Can you work these out from the model? Positions are in its coordinate system, mm. Face numbers are marked on the shaded views. A direction names the side the tool comes from. Coordinates: 2 decimals unless noted, no trailing zeros. Loops run counter-clockwise (first coordinate to the right, second up) from the corner with the lowest first, then second, coordinate; pieces in that order, holes last. Notation, with made-up numbers: M 15.25,-5.75 L 24.25,-5.75 A17 cw 24.25,13.25 Z; hole C 84,49 d9. An arc over 180 degrees is marked long. Answer as a JSON object with one key per item and string values. Group by question number.
Item 1: I'm going to push a flat-ended pin straight in: pin 1 Ø7 at (x, z) = (13, -0.5) entering from +Y. Where does the tip first touch, or does it pass through?
Item 2: Suppose I cut it at A-A (y = 19.54). Write out the boundary of the cut face in (x, z).
Item 3: Which directions (+Z, -Z, +X, -X, +Y, -Y) give clear straight access to the entire face, cutting with the end or side of a thin tool? Please do the marked faces 1 and 2.
Item 4: Suppose I cut it at B-B (x = 0). Write out the boundary of the cut face in (y, z).
Item 5: Suppose I cut it at D-D (y = 12). Write out the boundary of the cut face in (x, z), then the cut area to 3 significant figures.
Item 6: Suppose I cut it at C-C (y = 30.04). Count the separate pieces of the cut face and the enclosed holes in it, then the cut area to 3 significant figures.
Item 7: If I drill on line 1 (Z direction, x = -29, y = 30); line 2 (X direction, y = 12, z = -4.75); line 3 (Y direction, x = -11, z = -6), over which ranges is the centre line in solid material (lowest first)?
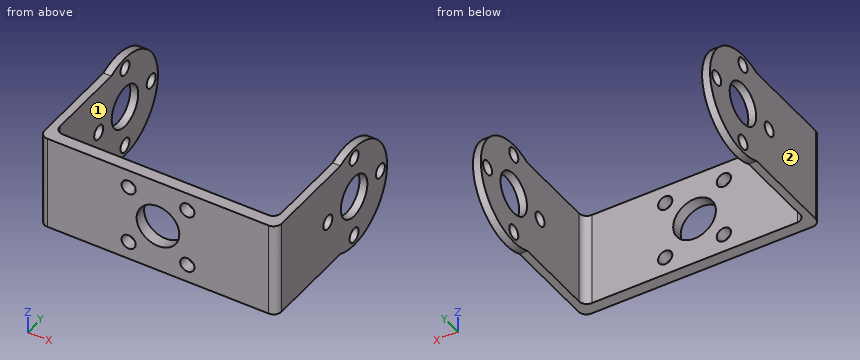
```python
from build123d import *

# Parameters (mm, degrees)
CROQUIS1_W              = 60
CROQUIS1_H              = 24
SALIENTE_EXTRUIR1_DEPTH = 2
CROQUIS3_R              = 5.3
SALIENTE_EXTRUIR2_DEPTH = 2
CROQUIS5_R              = 1.8
CORTAR_EXTRUIR1_DEPTH   = 2
CROQUIS6_W              = 60
CROQUIS6_H              = 24
SALIENTE_EXTRUIR3_DEPTH = 1
CORTAR_EXTRUIR2_REACH   = 46.22
CROQUIS7_R              = 5.4
CROQUIS7_R_2            = 1.8
REDONDEO1_R             = 2


with BuildPart() as part:
    # Croquis1 → Saliente-Extruir1 (new body)
    with BuildSketch(Plane(origin=(0, 0, 0), x_dir=(1, 0, 0), z_dir=(0, 1, 0))):
        Rectangle(CROQUIS1_W, CROQUIS1_H)
    extrude(amount=SALIENTE_EXTRUIR1_DEPTH)

    # Croquis3 → Saliente-Extruir2 (add)
    with BuildSketch(Plane(origin=(30, 0, 0), x_dir=(0, 0, -1), z_dir=(1, 0, 0))):
        with BuildLine():
            Line((12, 2), (-12, 2))
            Line((-12, 2), (-12, 24.589091819))
            ThreePointArc((-12, 24.589091819), (0, 43.22), (12, 24.589091819))
            Line((12, 24.589091819), (12, 2))
        make_face()
        with Locations((0, 30.04)):
            Circle(CROQUIS3_R, mode=Mode.SUBTRACT)
    saliente_extruir2 = extrude(amount=-SALIENTE_EXTRUIR2_DEPTH)

    # Croquis5 → Cortar-Extruir1 (cut)
    with BuildSketch(Plane(origin=(30, 0, 0), x_dir=(0, 0, -1), z_dir=(1, 0, 0))):
        with Locations((0, 40.54)):
            Circle(CROQUIS5_R)
        with Locations((10.5, 30.04)):
            Circle(CROQUIS5_R)
        with Locations((0, 19.54)):
            Circle(CROQUIS5_R)
        with Locations((-10.5, 30.04)):
            Circle(CROQUIS5_R)
    cortar_extruir1 = extrude(amount=-CORTAR_EXTRUIR1_DEPTH, mode=Mode.SUBTRACT)

    # Simetría1: Saliente-Extruir2, Cortar-Extruir1 across plane
    add(saliente_extruir2.mirror(Plane(origin=(0, 0, 0), x_dir=(0, 0, 1), z_dir=(1, 0, 0))))
    add(cortar_extruir1.mirror(Plane(origin=(0, 0, 0), x_dir=(0, 0, 1), z_dir=(1, 0, 0))), mode=Mode.SUBTRACT)

    # Croquis6 → Saliente-Extruir3 (add)
    with BuildSketch(Plane.XZ):
        Rectangle(CROQUIS6_W, CROQUIS6_H)
    extrude(amount=SALIENTE_EXTRUIR3_DEPTH)

    # Croquis7 → Cortar-Extruir2 (cut, up to next)
    with BuildSketch(Plane.XZ.offset(1), mode=Mode.PRIVATE) as cortar_extruir2_sk1:
        Circle(CROQUIS7_R)
    cortar_extruir2_tool1 = extrude(cortar_extruir2_sk1.sketch, amount=-CORTAR_EXTRUIR2_REACH, mode=Mode.PRIVATE) & part.part
    add(cortar_extruir2_tool1.solids().sort_by_distance((0, -1, 0))[0], mode=Mode.SUBTRACT)
    # Croquis7 → Cortar-Extruir2 (cut, up to next)
    with BuildSketch(Plane.XZ.offset(1), mode=Mode.PRIVATE) as cortar_extruir2_sk2:
        with Locations((7.424621202, -7.424621202)):
            Circle(CROQUIS7_R_2)
    cortar_extruir2_tool2 = extrude(cortar_extruir2_sk2.sketch, amount=-CORTAR_EXTRUIR2_REACH, mode=Mode.PRIVATE) & part.part
    add(cortar_extruir2_tool2.solids().sort_by_distance((7.424621, -1, -7.424621))[0], mode=Mode.SUBTRACT)
    # Croquis7 → Cortar-Extruir2 (cut, up to next)
    with BuildSketch(Plane.XZ.offset(1), mode=Mode.PRIVATE) as cortar_extruir2_sk3:
        with Locations((-7.423621202, -7.423621202)):
            Circle(CROQUIS7_R_2)
    cortar_extruir2_tool3 = extrude(cortar_extruir2_sk3.sketch, amount=-CORTAR_EXTRUIR2_REACH, mode=Mode.PRIVATE) & part.part
    add(cortar_extruir2_tool3.solids().sort_by_distance((-7.423621, -1, -7.423621))[0], mode=Mode.SUBTRACT)
    # Croquis7 → Cortar-Extruir2 (cut, up to next)
    with BuildSketch(Plane.XZ.offset(1), mode=Mode.PRIVATE) as cortar_extruir2_sk4:
        with Locations((-7.422621202, 7.424621202)):
            Circle(CROQUIS7_R_2)
    cortar_extruir2_tool4 = extrude(cortar_extruir2_sk4.sketch, amount=-CORTAR_EXTRUIR2_REACH, mode=Mode.PRIVATE) & part.part
    add(cortar_extruir2_tool4.solids().sort_by_distance((-7.422621, -1, 7.424621))[0], mode=Mode.SUBTRACT)
    # Croquis7 → Cortar-Extruir2 (cut, up to next)
    with BuildSketch(Plane.XZ.offset(1), mode=Mode.PRIVATE) as cortar_extruir2_sk5:
        with Locations((7.425621202, 7.423621202)):
            Circle(CROQUIS7_R_2)
    cortar_extruir2_tool5 = extrude(cortar_extruir2_sk5.sketch, amount=-CORTAR_EXTRUIR2_REACH, mode=Mode.PRIVATE) & part.part
    add(cortar_extruir2_tool5.solids().sort_by_distance((7.425621, -1, 7.423621))[0], mode=Mode.SUBTRACT)

    # Redondeo1
    redondeo1_edges = [part.edges().sort_by_distance(p)[0] for p in [
        (-28, 2, 0),
        (28, 2, 0),
        (-30, -1, 0),
        (30, -1, 0),
    ]]
    fillet(redondeo1_edges, radius=REDONDEO1_R)


solid = part.part
```
From the geometry:
{
 "1": {"pin 1": "y = 2"},
 "2": {"outline": "M -30,-12 L -28,-12 L -28,-1.8 L -30,-1.8 Z; M -30,1.8 L -28,1.8 L -28,12 L -30,12 Z; M 28,-12 L 30,-12 L 30,-1.8 L 28,-1.8 Z; M 28,1.8 L 30,1.8 L 30,12 L 28,12 Z"},
 "3": {"face 1": "+Z, -Z, +Y", "face 2": "+Z, -Z, -X, +Y, -Y"},
 "4": {"outline": "M -1,-12 L 2,-12 L 2,-5.4 L -1,-5.4 Z; M -1,5.4 L 2,5.4 L 2,12 L -1,12 Z"},
 "5": {"outline": "M -30,-12 L -28,-12 L -28,12 L -30,12 Z; M 28,-12 L 30,-12 L 30,12 L 28,12 Z", "area": "96.0 mm2"},
 "6": {"separate pieces": "8", "enclosed holes": "0", "area": "34.2 mm2"},
 "7": {"line 1": "-13.18 to -12.3, -8.7 to -5.3, 5.3 to 8.7, 12.3 to 13.18", "line 2": "-30 to -28, 28 to 30", "line 3": "-1 to 2"}
}
